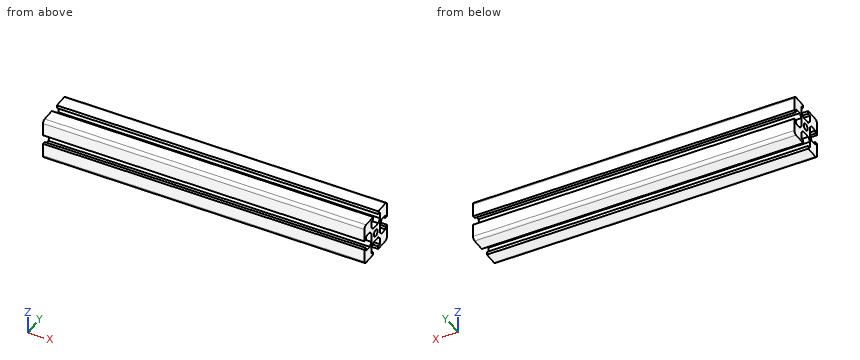
Autodesk Inventor part; units mm, degrees
ref_plane "YZ Plane" through (0, 0, 0) normal (1, 0, 0) x (0, 1, 0)
ref_plane "XZ Plane" through (0, 0, 0) normal (0, 1, 0) x (-1, 0, 0)
ref_plane "XY Plane" through (0, 0, 0) normal (0, 0, 1) x (1, 0, 0)
sketch "Sketch2" plane through (0, 0, 0) normal (1, 0, 0) x (0, 1, 0)
  line L0 (1.3843, 0) -> (1.397, 0)
  line L1 (17.653, 0) -> (11.684, 0)
  line L2 (11.684, 0) -> (11.684, -1.397)
  line L3 (11.684, -1.397) -> (13.1572, -1.397)
  line L4 (13.1572, -1.397) -> (13.1572, -4.5085)
  line L5 (13.1572, -4.5085) -> (11.7024, -5.9633)
  line L6 (11.7024, -5.9633) -> (7.3844, -5.9633)
  line L7 (7.3844, -5.9633) -> (5.9296, -4.5085)
  line L8 (5.9296, -4.5085) -> (5.9296, -1.397)
  line L9 (5.9296, -1.397) -> (7.4028, -1.397)
  line L10 (7.4028, -1.397) -> (7.4028, 0)
  line L11 (1.397, 0) -> (7.4028, 0)
  line L12 (11.684, 0) -> (19.05, 0)
  line L13 (5.9633, -7.3476) -> (5.9633, -11.6656)
  line L14 (4.5085, -5.8928) -> (5.9633, -7.3476)
  line L15 (5.9633, -11.6656) -> (4.5085, -13.1204)
  line L16 (1.397, -13.1204) -> (1.397, -11.6472)
  line L17 (4.5085, -13.1204) -> (1.397, -13.1204)
  line L18 (1.397, -11.6472) -> (0, -11.6472)
  line L19 (1.397, -5.8928) -> (4.5085, -5.8928)
  line L20 (0, -7.366) -> (1.397, -7.366)
  line L21 (1.397, -7.366) -> (1.397, -5.8928)
  line L22 (7.3476, -13.0867) -> (11.6656, -13.0867)
  line L23 (5.8928, -14.5415) -> (7.3476, -13.0867)
  line L24 (11.6656, -13.0867) -> (13.1204, -14.5415)
  line L25 (13.1204, -17.653) -> (11.6472, -17.653)
  line L26 (13.1204, -14.5415) -> (13.1204, -17.653)
  line L27 (11.6472, -17.653) -> (11.6472, -19.05)
  line L28 (5.8928, -17.653) -> (5.8928, -14.5415)
  line L29 (7.366, -19.05) -> (7.366, -17.653)
  line L30 (7.366, -17.653) -> (5.8928, -17.653)
  line L31 (13.0867, -11.7024) -> (13.0867, -7.3844)
  line L32 (14.5415, -13.1572) -> (13.0867, -11.7024)
  line L33 (13.0867, -7.3844) -> (14.5415, -5.9296)
  line L34 (17.653, -5.9296) -> (17.653, -7.4028)
  line L35 (14.5415, -5.9296) -> (17.653, -5.9296)
  line L36 (17.653, -7.4028) -> (19.05, -7.4028)
  line L37 (17.653, -13.1572) -> (14.5415, -13.1572)
  line L38 (19.05, -11.684) -> (17.653, -11.684)
  line L39 (17.653, -11.684) -> (17.653, -13.1572)
  line L40 (1.3843, 0) -> (1.397, 0)
  line L41 (19.05, -1.397) -> (19.05, -7.4028)
  line L42 (19.05, -11.684) -> (19.05, -17.653)
  line L43 (17.653, -19.05) -> (11.6472, -19.05)
  line L44 (7.366, -19.05) -> (1.397, -19.05)
  line L45 (0, -17.653) -> (0, -11.6472)
  line L46 (0, -7.366) -> (0, -1.397)
  line L47 (0, -7.366) -> (0, -1.397)
  circle A0 centre (9.525, -9.525) radius 1.5875
  line L48 (1.3843, 0) -> (1.397, 0)
  line L49 (0, -1.397) -> (0, -1.3843)
  arc A1 (1.397, 0) -> (0, -1.397) centre (1.397, -1.397) ccw
  arc A2 (0, -17.653) -> (1.397, -19.05) centre (1.397, -17.653) ccw
  arc A3 (17.653, -19.05) -> (19.05, -17.653) centre (17.653, -17.653) ccw
  arc A4 (19.05, -1.397) -> (17.653, 0) centre (17.653, -1.397) ccw
  point P0 (0, 0)
  dimension "d34" = 7.366
  dimension "d35" = 1.397
  dimension "d37" = 1.4732
  dimension "d38" = 3.1115
  dimension "d39" = 2.0574
  dimension "d40" = 135
  dimension "d41" = 4.318
  dimension "d42" = 2.0574
  dimension "d43" = 1.4732
  dimension "d46" = 1.397
  dimension "d49" = 360
  dimension "d56" = 19.05
  dimension "d58" = 3.175
  dimension "d61" = 1.397
  dimension "d62" = 1.397
  dimension "d63" = 1.397
  dimension "d64" = 1.397
  dimension "d67" = 360
  dimension "d71" = 3.1115
extrude "Extrusion1" add sketch "Sketch2" along normal blind 147.32
properties part number "Extrusion"
Here's how the part is built. I have some questions about the finished solid (model axes, mm). Coordinates: 2 decimals unless noted, no trailing zeros. Write each loop counter-clockwise with the first axis right and the second up, starting at its lowest first coordinate (ties: lowest second). Pieces come first, ordered by that corner, then holes.
1) If I drill on line 1 (Y direction, x = 83.5, z = -4.5); line 2 (Z direction, x = 126.5, y = 17.75); line 3 (Y direction, x = 126, z = -12.75), over which ranges is the centre line in solid material (lowest first)?
Filled in:
line 1: y = 0 to 5.93, 13.16 to 19.05
line 2: z = -19.05 to -11.68, -7.4 to 0
line 3: y = 0 to 1.4, 4.88 to 14.13, 17.65 to 19.05
2) If we section it at B-B (z = -2.75): List the corners of the cut face in (x, y) for me, plus the area to 3 significant figures.
Filled in:
outline: (0, 0) - (147.32, 0) - (147.32, 5.93) - (0, 5.93) - close; (0, 13.16) - (147.32, 13.16) - (147.32, 19.05) - (0, 19.05) - close
area: 1,740 mm2
3) I'm going to push flat-ended pins straight in: pin 1 (1.9 mm diameter, centred on y = 9.525, z = -9.525, fed in from +X); pin 2 (3.5 mm diameter, centred on x = 57, y = 9.5, fed in from -Z); pin 3 (1.5 mm diameter, centred on x = 88.5, z = -18.5, fed in from -Y); pin 4 (4 mm diameter, centred on x = 36.5, y = 9.5, fed in from +Z). Where does each tip first touch, or does it pass through?
Filled in:
pin 1: passes through
pin 2: stops at z = -13.09
pin 3: stops at y = 0
pin 4: stops at z = -5.96
4) If we section it at A-A (y = 15.75): List the corners of the cut face in (x, z) for me, plus the area to 3 significant figures.
Filled in:
outline: (0, -19.05) - (147.32, -19.05) - (147.32, -13.16) - (0, -13.16) - close; (0, -5.93) - (147.32, -5.93) - (147.32, 0) - (0, 0) - close
area: 1,740 mm2
